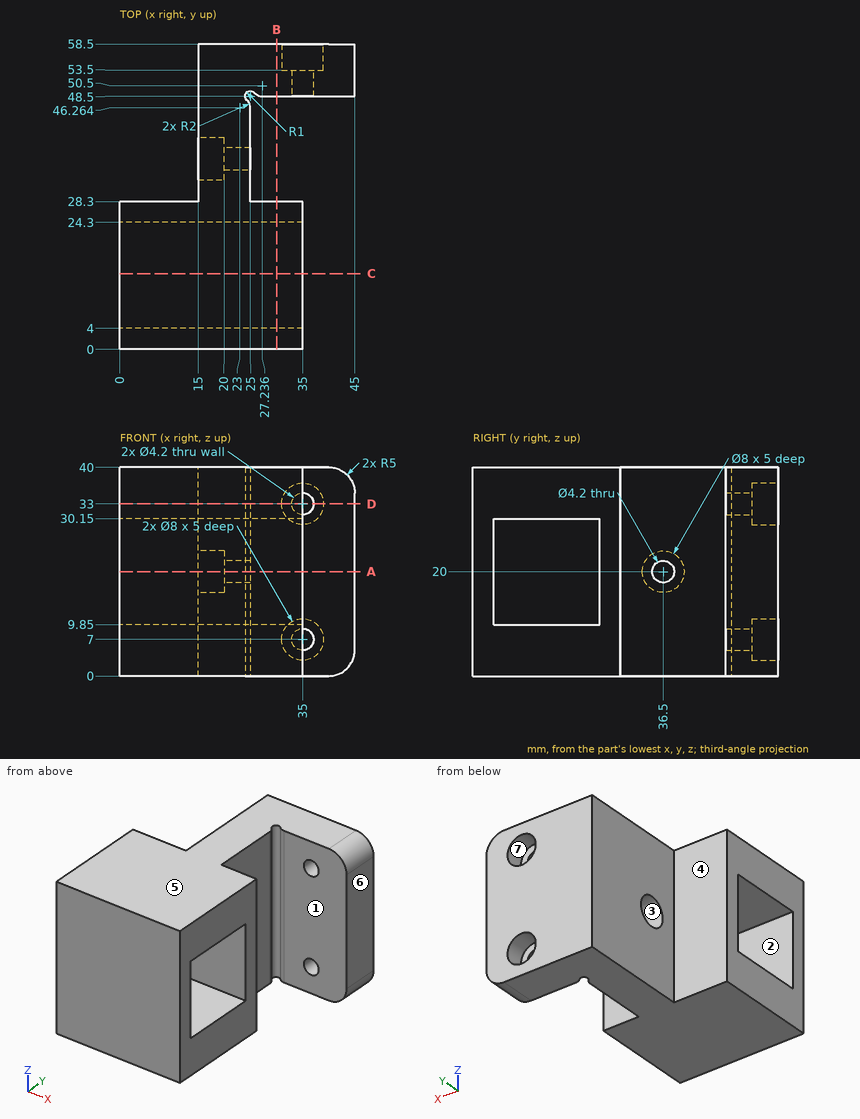
Design review of the part shown in the three views and the two pictorial views. Dimensions are in mm from the part's minimum x, y and z. A direction names the side the tool comes from. Round coordinates to 2 decimals unless told otherwise and drop trailing zeros. Loops run counter-clockwise (first coordinate to the right, second up) from the corner with the lowest first, then second, coordinate; pieces in that order, holes last. Notation, with made-up numbers: M -2.5,67.25 L 26.5,67.25 A12 cw 26.5,71.25 Z; hole C 8.25,35.5 d4. An arc over 180 degrees is marked long. Write item = value, one per line.
Item 1: Take a section at A-A on z = 20. Write out the cut boundary in (x, y), then the cut area to 3 significant figures.
Return value:
outline = M 0,0 L 35,0 L 35,4 L 0,4 Z; M 0,24.3 L 35,24.3 L 35,28.3 L 25,28.3 L 25,34.4 L 20,34.4 L 20,32.5 L 15,32.5 L 15,28.3 L 0,28.3 Z; M 15,40.5 L 20,40.5 L 20,38.6 L 25,38.6 L 25,46.26 A2 ccw 24.33,47.75 A1 cw long 25.75,49.17 A2 ccw 27.24,48.5 L 45,48.5 L 45,58.5 L 15,58.5 Z
area = 718 mm2
Item 2: Machinability: for the marked faces 1, 2, 3 and 4, which of the approach directions +Z, -Z, +X, -X, +Y, -Y give a long, thin tool a straight path to every point of the face, cutting with its end or side? Answer none if there is none.
Return value:
face_1 = +Z, -Z, +X
face_2 = +X, -X
face_3 = -X
face_4 = +Z, -Z, -X, +Y
Item 3: The part is to be moulded in two halves that separate along Z. For the marked faces 5, 6 and 7, say which applies: released by +Z, released by -Z, zero draft, split by the parting line, or undercut.
Return value:
face_5 = released by +Z
face_6 = zero draft
face_7 = undercut
Item 4: Take a section at D-D on z = 33. Write out the cut boundary in (x, y), then the cut area to 3 significant figures.
Return value:
outline = M 0,0 L 35,0 L 35,28.3 L 25,28.3 L 25,46.26 A2 ccw 24.33,47.75 A1 cw long 25.75,49.17 A2 ccw 27.24,48.5 L 32.9,48.5 L 32.9,53.5 L 31,53.5 L 31,58.5 L 15,58.5 L 15,28.3 L 0,28.3 Z; M 37.1,48.5 L 45,48.5 L 45,58.5 L 39,58.5 L 39,53.5 L 37.1,53.5 Z
area = 1,430 mm2
Item 5: Take a section at B-B on x = 30. Write out the cut boundary in (y, z), then the cut area to 3 significant figures.
Return value:
outline = M 0,0 L 28.3,0 L 28.3,40 L 0,40 Z; M 48.5,0 L 58.5,0 L 58.5,40 L 48.5,40 Z; hole M 4,9.85 L 24.3,9.85 L 24.3,30.15 L 4,30.15 Z
area = 1,120 mm2
Item 6: Insertion check: P1, Ø2.5, axis at y = 37, z = 18, coming from the -X side; P2, Ø13, axis at y = 36.5, z = 20, coming from the -X side; P3, Ø1, axis at y = 23.5, z = 13, coming from the +X side; P4, Ø22.5, axis at y = 8, z = 19, coming from the +X side. Each pin has a flat end and moves straight along its axis. Give the tip position at first contact, or say it passes through.
Return value:
P1 = 20
P2 = 15
P3 = through
P4 = 35
Item 7: For line 1 (Z direction, x = 35, y = 55.85); line 2 (Z direction, x = 35, y = 50); line 3 (Y direction, x = 34, z = 16), list the stretches that pass through material, from the lowest coordinate up. Write a range as [from, to].
Return value:
line_1 = [0, 3], [11, 29], [37, 40]
line_2 = [0, 4.9], [9.1, 30.9], [35.1, 40]
line_3 = [0, 4], [24.3, 28.3], [48.5, 58.5]
Item 8: Take a section at C-C on y = 14.5. Write out the cut boundary in (x, z).
Return value:
outline = M 0,0 L 35,0 L 35,9.85 L 0,9.85 Z; M 0,30.15 L 35,30.15 L 35,40 L 0,40 Z
